For this review, take the finished solid that the model builds, in its own axes (mm). Round coordinates to 2 decimals unless told otherwise and drop trailing zeros. Order: outer loops, then holes, each group sorted by start corner. A loop starts at its lowest first (then second) coordinate and runs counter-clockwise, first axis right, second up.
```python
from build123d import *

# Parameters (mm, degrees)
SKETCH1_W           = 110
SKETCH1_H           = 100
SKETCH1_R           = 1.6
SKETCH1_R_2         = 1.35
BOSS_EXTRUDE1_DEPTH = 3
SKETCH2_R           = 10
SKETCH2_R_2         = 1.6
CUT_EXTRUDE1_DEPTH  = 4
CUT_EXTRUDE2_DEPTH  = 4
FILLET2_R           = 3
CUT_EXTRUDE_1_DEPTH = 4


with BuildPart() as part:
    # Sketch1 → Boss-Extrude1 (new body)
    with BuildSketch(Plane(origin=(0, 0, 0), x_dir=(1, 0, 0), z_dir=(0, 1, 0))):
        Rectangle(SKETCH1_W, SKETCH1_H)
        with Locations((42.5, 41.5)):
            Circle(SKETCH1_R, mode=Mode.SUBTRACT)
        with Locations((20, 35)):
            Circle(SKETCH1_R_2, mode=Mode.SUBTRACT)
        with Locations((-20, 35)):
            Circle(SKETCH1_R_2, mode=Mode.SUBTRACT)
        with Locations((28, -35)):
            Circle(SKETCH1_R_2, mode=Mode.SUBTRACT)
        with Locations((-28, -35)):
            Circle(SKETCH1_R_2, mode=Mode.SUBTRACT)
        with Locations((-42.5, 41.5)):
            Circle(SKETCH1_R, mode=Mode.SUBTRACT)
        with Locations((42.5, -41.5)):
            Circle(SKETCH1_R, mode=Mode.SUBTRACT)
        with Locations((-42.5, -41.5)):
            Circle(SKETCH1_R, mode=Mode.SUBTRACT)
    extrude(amount=BOSS_EXTRUDE1_DEPTH)

    # Sketch2 → Cut-Extrude1 (cut, through all)
    with BuildSketch(Plane(origin=(0, 3, 0), x_dir=(1, 0, 0), z_dir=(0, 1, 0))):
        Circle(SKETCH2_R)
        with Locations((-10.429825023, -10.429825023)):
            Circle(SKETCH2_R_2)
        with Locations((10.429825023, -10.429825023)):
            Circle(SKETCH2_R_2)
        with Locations((-10.429825023, 10.429825023)):
            Circle(SKETCH2_R_2)
        with Locations((10.429825023, 10.429825023)):
            Circle(SKETCH2_R_2)
        with Locations((25.5, 0)):
            Circle(SKETCH2_R_2)
        with Locations((0, -25.5)):
            Circle(SKETCH2_R_2)
        with Locations((-25.5, 0)):
            Circle(SKETCH2_R_2)
        with Locations((0, 25.5)):
            Circle(SKETCH2_R_2)
        with BuildLine():
            Line((-14, 21.6), (14, 21.6))
            ThreePointArc((14, 21.6), (15.6, 20), (14, 18.4))
            Line((14, 18.4), (-14, 18.4))
            ThreePointArc((-14, 18.4), (-15.6, 20), (-14, 21.6))
        make_face()
        with BuildLine():
            Line((-14, -21.6), (14, -21.6))
            ThreePointArc((14, -21.6), (15.6, -20), (14, -18.4))
            Line((14, -18.4), (-14, -18.4))
            ThreePointArc((-14, -18.4), (-15.6, -20), (-14, -21.6))
        make_face()
        with BuildLine():
            Line((21.6, 14), (21.6, -14))
            ThreePointArc((21.6, -14), (20, -15.6), (18.4, -14))
            Line((18.4, -14), (18.4, 14))
            ThreePointArc((18.4, 14), (20, 15.6), (21.6, 14))
        make_face()
        with BuildLine():
            Line((-21.6, 14), (-21.6, -14))
            ThreePointArc((-21.6, -14), (-20, -15.6), (-18.4, -14))
            Line((-18.4, -14), (-18.4, 14))
            ThreePointArc((-18.4, 14), (-20, 15.6), (-21.6, 14))
        make_face()
        with BuildLine():
            Line((-20.36862915, 22.63137085), (-16.89985207, 19.16259377))
            ThreePointArc((-16.89985207, 19.16259377), (-16.89985207, 16.89985207), (-19.16259377, 16.89985207))
            Line((-19.16259377, 16.89985207), (-22.63137085, 20.36862915))
            ThreePointArc((-22.63137085, 20.36862915), (-22.63137085, 22.63137085), (-20.36862915, 22.63137085))
        make_face()
        with BuildLine():
            Line((20.36862915, 22.63137085), (16.89985207, 19.16259377))
            ThreePointArc((16.89985207, 19.16259377), (16.89985207, 16.89985207), (19.16259377, 16.89985207))
            Line((19.16259377, 16.89985207), (22.63137085, 20.36862915))
            ThreePointArc((22.63137085, 20.36862915), (22.63137085, 22.63137085), (20.36862915, 22.63137085))
        make_face()
        with BuildLine():
            Line((20.36862915, -22.63137085), (16.89985207, -19.16259377))
            ThreePointArc((16.89985207, -19.16259377), (16.89985207, -16.89985207), (19.16259377, -16.89985207))
            Line((19.16259377, -16.89985207), (22.63137085, -20.36862915))
            ThreePointArc((22.63137085, -20.36862915), (22.63137085, -22.63137085), (20.36862915, -22.63137085))
        make_face()
        with BuildLine():
            Line((-20.36862915, -22.63137085), (-16.89985207, -19.16259377))
            ThreePointArc((-16.89985207, -19.16259377), (-16.89985207, -16.89985207), (-19.16259377, -16.89985207))
            Line((-19.16259377, -16.89985207), (-22.63137085, -20.36862915))
            ThreePointArc((-22.63137085, -20.36862915), (-22.63137085, -22.63137085), (-20.36862915, -22.63137085))
        make_face()
    extrude(amount=-CUT_EXTRUDE1_DEPTH, mode=Mode.SUBTRACT)

    # Sketch3 → Cut-Extrude2 (cut, through all)
    with BuildSketch(Plane(origin=(0, 3, 0), x_dir=(1, 0, 0), z_dir=(0, 1, 0))):
        with BuildLine():
            Line((3.606244584, 33.656497116), (8.555992052, 28.706749647))
            ThreePointArc((8.555992052, 28.706749647), (8.555992052, 26.444007948), (6.293250353, 26.444007948))
            Line((6.293250353, 26.444007948), (1.343502884, 31.393755416))
            ThreePointArc((1.343502884, 31.393755416), (1.343502884, 33.656497116), (3.606244584, 33.656497116))
        make_face()
        with BuildLine():
            Line((-1.343502884, 31.393755416), (-6.293250353, 26.444007948))
            ThreePointArc((-6.293250353, 26.444007948), (-8.555992052, 26.444007948), (-8.555992052, 28.706749647))
            Line((-8.555992052, 28.706749647), (-3.606244584, 33.656497116))
            ThreePointArc((-3.606244584, 33.656497116), (-1.343502884, 33.656497116), (-1.343502884, 31.393755416))
        make_face()
        with BuildLine():
            Line((-3.606244584, 36.343502884), (-8.555992052, 41.293250353))
            ThreePointArc((-8.555992052, 41.293250353), (-8.555992052, 43.555992052), (-6.293250353, 43.555992052))
            Line((-6.293250353, 43.555992052), (-1.343502884, 38.606244584))
            ThreePointArc((-1.343502884, 38.606244584), (-1.343502884, 36.343502884), (-3.606244584, 36.343502884))
        make_face()
        with BuildLine():
            Line((1.343502884, 38.606244584), (6.293250353, 43.555992052))
            ThreePointArc((6.293250353, 43.555992052), (8.555992052, 43.555992052), (8.555992052, 41.293250353))
            Line((8.555992052, 41.293250353), (3.606244584, 36.343502884))
            ThreePointArc((3.606244584, 36.343502884), (1.343502884, 36.343502884), (1.343502884, 38.606244584))
        make_face()
        with BuildLine():
            Line((11.6, 38.5), (11.6, 31.5))
            ThreePointArc((11.6, 31.5), (10, 29.9), (8.4, 31.5))
            Line((8.4, 31.5), (8.4, 38.5))
            ThreePointArc((8.4, 38.5), (10, 40.1), (11.6, 38.5))
        make_face()
        with BuildLine():
            Line((-11.6, 38.5), (-11.6, 31.5))
            ThreePointArc((-11.6, 31.5), (-10, 29.9), (-8.4, 31.5))
            Line((-8.4, 31.5), (-8.4, 38.5))
            ThreePointArc((-8.4, 38.5), (-10, 40.1), (-11.6, 38.5))
        make_face()
        with BuildLine():
            Line((3.606244584, -33.656497116), (8.555992052, -28.706749647))
            ThreePointArc((8.555992052, -28.706749647), (8.555992052, -26.444007948), (6.293250353, -26.444007948))
            Line((6.293250353, -26.444007948), (1.343502884, -31.393755416))
            ThreePointArc((1.343502884, -31.393755416), (1.343502884, -33.656497116), (3.606244584, -33.656497116))
        make_face()
        with BuildLine():
            Line((11.6, -38.5), (11.6, -31.5))
            ThreePointArc((11.6, -31.5), (10, -29.9), (8.4, -31.5))
            Line((8.4, -31.5), (8.4, -38.5))
            ThreePointArc((8.4, -38.5), (10, -40.1), (11.6, -38.5))
        make_face()
        with BuildLine():
            Line((1.343502884, -38.606244584), (6.293250353, -43.555992052))
            ThreePointArc((6.293250353, -43.555992052), (8.555992052, -43.555992052), (8.555992052, -41.293250353))
            Line((8.555992052, -41.293250353), (3.606244584, -36.343502884))
            ThreePointArc((3.606244584, -36.343502884), (1.343502884, -36.343502884), (1.343502884, -38.606244584))
        make_face()
        with BuildLine():
            Line((-1.343502884, -31.393755416), (-6.293250353, -26.444007948))
            ThreePointArc((-6.293250353, -26.444007948), (-8.555992052, -26.444007948), (-8.555992052, -28.706749647))
            Line((-8.555992052, -28.706749647), (-3.606244584, -33.656497116))
            ThreePointArc((-3.606244584, -33.656497116), (-1.343502884, -33.656497116), (-1.343502884, -31.393755416))
        make_face()
        with BuildLine():
            Line((-11.6, -38.5), (-11.6, -31.5))
            ThreePointArc((-11.6, -31.5), (-10, -29.9), (-8.4, -31.5))
            Line((-8.4, -31.5), (-8.4, -38.5))
            ThreePointArc((-8.4, -38.5), (-10, -40.1), (-11.6, -38.5))
        make_face()
        with BuildLine():
            Line((-3.606244584, -36.343502884), (-8.555992052, -41.293250353))
            ThreePointArc((-8.555992052, -41.293250353), (-8.555992052, -43.555992052), (-6.293250353, -43.555992052))
            Line((-6.293250353, -43.555992052), (-1.343502884, -38.606244584))
            ThreePointArc((-1.343502884, -38.606244584), (-1.343502884, -36.343502884), (-3.606244584, -36.343502884))
        make_face()
        with BuildLine():
            Line((-56, 45), (-41, 30))
            ThreePointArc((-41, 30), (-28.573593129, 0), (-41, -30))
            Line((-41, -30), (-56, -45))
            Line((-56, -45), (-56, 45))
        make_face()
        with BuildLine():
            Line((56, 45), (41, 30))
            ThreePointArc((41, 30), (28.573593129, 0), (41, -30))
            Line((41, -30), (56, -45))
            Line((56, -45), (56, 45))
        make_face()
    extrude(amount=-CUT_EXTRUDE2_DEPTH, mode=Mode.SUBTRACT)

    # Fillet2
    fillet2_edges = [part.edges().sort_by_distance(p)[0] for p in [
        (-55, 1.5, 44),
        (-55, 1.5, -44),
        (55, 1.5, 44),
        (55, 1.5, -44),
        (55, 1.5, 50),
        (-55, 1.5, 50),
        (-55, 1.5, -50),
        (55, 1.5, -50),
    ]]
    fillet(fillet2_edges, radius=FILLET2_R)

    # 草图1 → 切除-拉伸1 (cut, through all)
    with BuildSketch(Plane(origin=(0, 3, 0), x_dir=(1, 0, 0), z_dir=(0, 1, 0))):
        with BuildLine():
            Line((-27.85, -41), (-27.85, -44))
            ThreePointArc((-27.85, -44), (-29.7, -45.85), (-31.55, -44))
            Line((-31.55, -44), (-31.55, -41))
            ThreePointArc((-31.55, -41), (-29.7, -39.15), (-27.85, -41))
        make_face()
        with BuildLine():
            Line((27.85, -41), (27.85, -44))
            ThreePointArc((27.85, -44), (29.7, -45.85), (31.55, -44))
            Line((31.55, -44), (31.55, -41))
            ThreePointArc((31.55, -41), (29.7, -39.15), (27.85, -41))
        make_face()
        with BuildLine():
            Line((27.85, 41), (27.85, 44))
            ThreePointArc((27.85, 44), (29.7, 45.85), (31.55, 44))
            Line((31.55, 44), (31.55, 41))
            ThreePointArc((31.55, 41), (29.7, 39.15), (27.85, 41))
        make_face()
        with BuildLine():
            Line((-27.85, 41), (-27.85, 44))
            ThreePointArc((-27.85, 44), (-29.7, 45.85), (-31.55, 44))
            Line((-31.55, 44), (-31.55, 41))
            ThreePointArc((-31.55, 41), (-29.7, 39.15), (-27.85, 41))
        make_face()
    extrude(amount=-CUT_EXTRUDE_1_DEPTH, mode=Mode.SUBTRACT)


solid = part.part
```
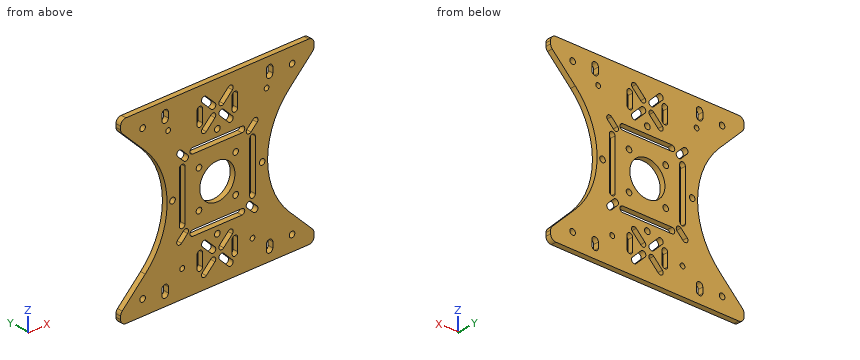
Q1. Clearance check with flat-ended pins moving along their axes: pin 1 (4 mm diameter, centred on x = 25.5, z = 0, fed in from +Y); pin 2 (1.5 mm diameter, centred on y = 2.5, z = -18, fed in from -X); pin 3 (1.5 mm diameter, centred on y = 1, z = 42.5, fed in from -X); pin 4 (0.9 mm diameter, centred on y = 1.5, z = 42.5, fed in from +X). State where each tip first meets the part, or that it passes through.
Q2. Take a section at A-A, the plane x = -42.5. State the section outline as (y, z) points.
Q3. Take a section at C-C, the plane y = 1.05. Count the separate pieces of the cut face and the enclosed holes in it, plus the area to 3 significant figures.
Q4. Wall thickness on line 1 (Z direction, x = 25.5, y = 0.85); line 2 (X direction, y = 1.7, z = 32); line 3 (Z direction, x = 0, y = 2.05): over which ranges is each line inside the solid? List them lowest first.
Q5. Take a section at B-B, the plane z = 0. State the section outline as (x, y) points.
Working result:
1. pin 1: stops at y = 3
1. pin 2: stops at x = -32.94
1. pin 3: stops at x = -54.24
1. pin 4: stops at x = 53.95
2. outline: (0, -50) - (3, -50) - (3, -43.1) - (0, -43.1) - close; (0, -39.9) - (3, -39.9) - (3, -31.5) - (0, -31.5) - close; (0, 31.5) - (3, 31.5) - (3, 39.9) - (0, 39.9) - close; (0, 43.1) - (3, 43.1) - (3, 50) - (0, 50) - close
3. separate pieces: 1
3. enclosed holes: 41
3. area: 6,520 mm2
4. line 1: z = -50 to -1.6, 1.6 to 50
4. line 2: x = -43 to -11.6, -8.4 to -5.26, -0.96 to 0.96, 5.26 to 8.4, 11.6 to 43
4. line 3: z = -50 to -27.1, -23.9 to -21.6, -18.4 to -10, 10 to 18.4, 21.6 to 23.9, 27.1 to 50
5. outline: (-28.57, 0) - (-27.1, 0) - (-27.1, 3) - (-28.57, 3) - close; (-23.9, 0) - (-21.6, 0) - (-21.6, 3) - (-23.9, 3) - close; (-18.4, 0) - (-10, 0) - (-10, 3) - (-18.4, 3) - close; (10, 0) - (18.4, 0) - (18.4, 3) - (10, 3) - close; (21.6, 0) - (23.9, 0) - (23.9, 3) - (21.6, 3) - close; (27.1, 0) - (28.57, 0) - (28.57, 3) - (27.1, 3) - close
